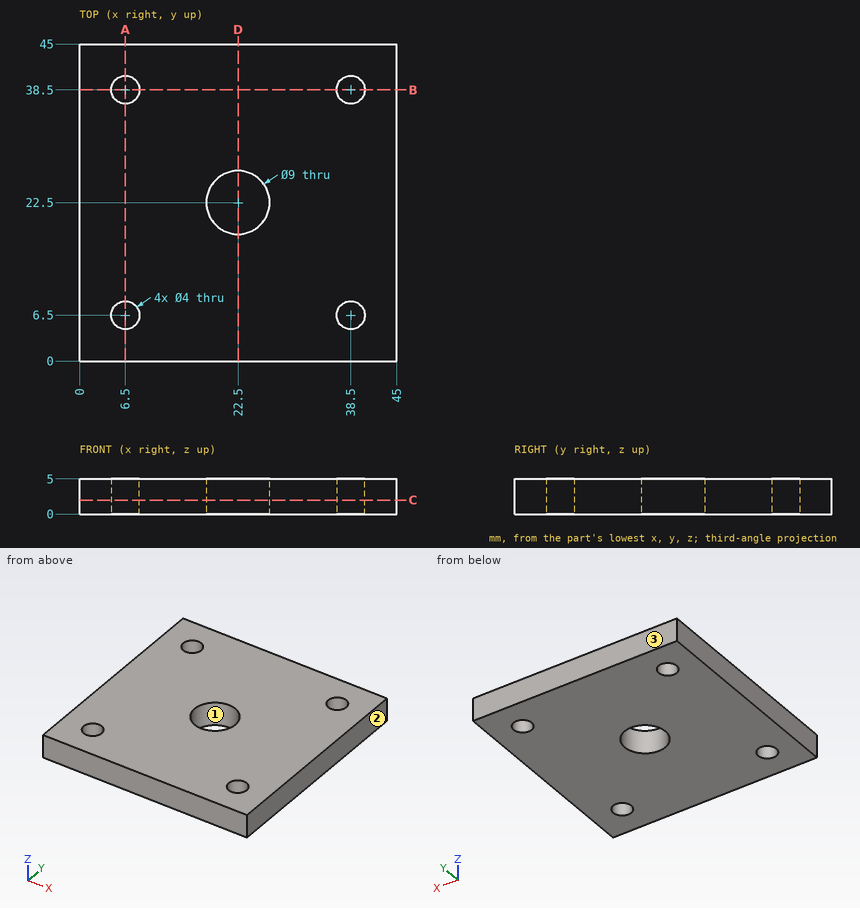
For this review, use the dimensioned drawing (mm, ordinates from the lowest corner) and the shaded views. Round coordinates to 2 decimals unless told otherwise and drop trailing zeros. Write each loop counter-clockwise with the first axis right and the second up, starting at its lowest first coordinate (ties: lowest second). Pieces come first, ordered by that corner, then holes. Notation, with made-up numbers: M 57,68 L 75,68 A13 ccw 75,86 Z; hole C 58,-17 d5. An arc over 180 degrees is marked long. Use CSV: the item, a comma, the result in double quotes. Start each with the question number.
(1) We need section C-C, the plane z = 2. State the section outline as (x, y) points.
(2) We need section A-A, the plane x = 6.5. State the section outline as (y, z) points, then the cut area to 3 significant figures.
(3) For line 1 along X through (y, z) = (6.5, 2.7); line 2 along X through (y, z) = (39, 3.5), list the stretches that pass through material, from the lowest coordinate up.
(4) We need section D-D, the plane x = 22.5. State the section outline as (y, z) points.
(5) The part is to be moulded in two halves that separate along Y. For the marked faces 1, 2 and 3, say which applies: +Y half, -Y half, draft (parallel to the pull), parting line (faces both ways), or undercut.
Findings:
1,outline,"M 0,0 L 45,0 L 45,45 L 0,45 Z; hole C 6.5,6.5 d4; hole C 6.5,38.5 d4; hole C 22.5,22.5 d9; hole C 38.5,6.5 d4; hole C 38.5,38.5 d4"
2,outline,"M 0,0 L 4.5,0 L 4.5,5 L 0,5 Z; M 8.5,0 L 36.5,0 L 36.5,5 L 8.5,5 Z; M 40.5,0 L 45,0 L 45,5 L 40.5,5 Z"
2,area,"185 mm^2"
3,line 1,"0 to 4.5, 8.5 to 36.5, 40.5 to 45"
3,line 2,"0 to 4.56, 8.44 to 36.56, 40.44 to 45"
4,outline,"M 0,0 L 18,0 L 18,5 L 0,5 Z; M 27,0 L 45,0 L 45,5 L 27,5 Z"
5,face 1,"undercut"
5,face 2,"draft"
5,face 3,"+Y half"
